from build123d import *

# Parameters (mm, degrees)
F0_W      = 228.6
F0_H      = 228.6
F1_DEPTH  = 38.1
F2_W      = 152.4
F2_H      = 152.4
F3_DEPTH  = 38.1
F4_W      = 38.1
F4_H      = 38.1
F5_DEPTH  = 1143
F6_W      = 228.6
F6_H      = 228.6
F7_DEPTH  = 38.1
F8_W      = 152.4
F8_H      = 152.4
F9_DEPTH  = 38.1
F10_W     = 38.1
F10_H     = 38.1
F11_DEPTH = 342.9
F12_W     = 38.1
F12_H     = 38.1
F13_DEPTH = 342.9
F14_R     = 6.35
F15_DEPTH = 0.254
F16_R     = 6.35
F17_DEPTH = 0.254
F18_R     = 6.35
F19_DEPTH = 0.254


with BuildPart() as f1:
    # F0 (on Top) → F1 (new body)
    with BuildSketch(Plane.XY):
        Rectangle(F0_W, F0_H)
    extrude(amount=-F1_DEPTH)

    # F2 (on face) → F3 (cut)
    with BuildSketch(Plane.XY):
        Rectangle(F2_W, F2_H)
    extrude(amount=-F3_DEPTH, mode=Mode.SUBTRACT)

    # F4 (on face) → F5 (join)
    with BuildSketch(Plane.XY):
        with Locations((-95.25, 95.25)):
            Rectangle(F4_W, F4_H)
        with Locations((95.25, 95.25)):
            Rectangle(F4_W, F4_H)
        with Locations((95.25, -95.25)):
            Rectangle(F4_W, F4_H)
        with Locations((-95.25, -95.25)):
            Rectangle(F4_W, F4_H)
    extrude(amount=F5_DEPTH)

    # F6 (on face) → F7 (join)
    with BuildSketch(Plane.XY.offset(1143)):
        Rectangle(F6_W, F6_H)
    extrude(amount=F7_DEPTH)

    # F8 (on face) → F9 (cut)
    with BuildSketch(Plane.XY.offset(1181.1)):
        Rectangle(F8_W, F8_H)
    extrude(amount=-F9_DEPTH, mode=Mode.SUBTRACT)

    # F10 (on face) → F11 (join)
    with BuildSketch(Plane(origin=(0, 0, 1143), x_dir=(1, 0, 0), z_dir=(0, 0, -1))):
        with Locations((95.25, 57.15)):
            Rectangle(F10_W, F10_H)
        with Locations((95.25, -57.15)):
            Rectangle(F10_W, F10_H)
    extrude(amount=F11_DEPTH)

    # F12 (on face) → F13 (join)
    with BuildSketch(Plane(origin=(0, 0, 1143), x_dir=(1, 0, 0), z_dir=(0, 0, -1))):
        with Locations((-95.25, -57.15)):
            Rectangle(F12_W, F12_H)
        with Locations((-95.25, 57.15)):
            Rectangle(F12_W, F12_H)
    extrude(amount=F13_DEPTH)

    # F14 (on face) → F15 (join)
    with BuildSketch(Plane(origin=(-114.3, 0, 0), x_dir=(0, -1, 0), z_dir=(-1, 0, 0))):
        with Locations((-95.25, -19.05)):
            Circle(F14_R)
        with Locations((95.25, -19.05)):
            Circle(F14_R)
    extrude(amount=F15_DEPTH)

    # F16 (on face) → F17 (cut)
    with BuildSketch(Plane.YZ.offset(-76.2)):
        with Locations((-57.15, 819.15)):
            Circle(F16_R)
        with Locations((57.15, 819.15)):
            Circle(F16_R)
    extrude(amount=-F17_DEPTH, mode=Mode.SUBTRACT)

    # F18 (on face) → F19 (cut)
    with BuildSketch(Plane(origin=(76.2, 0, 0), x_dir=(0, -1, 0), z_dir=(-1, 0, 0))):
        with Locations((-57.15, 819.15)):
            Circle(F18_R)
        with Locations((57.15, 819.15)):
            Circle(F18_R)
    extrude(amount=-F19_DEPTH, mode=Mode.SUBTRACT)


solid = f1.part
Verification items for the finished model (mm, model axes). A direction names the side the tool comes from. Coordinates: 2 decimals unless noted, no trailing zeros. Write each loop counter-clockwise with the first axis right and the second up, starting at its lowest first coordinate (ties: lowest second). Pieces come first, ordered by that corner, then holes. Notation, with made-up numbers: M 38.25,42 L 84.25,42 A29 cw 84.25,80 Z; hole C 43.25,69 d8. An arc over 180 degrees is marked long. Use a Markdown table: item, result.
Q1. Set-up check for faces 4 (the face through (95, 76.2, 394)), 5 (the face through (-1, -95, 0)), 6 (the face through (76.2, -1, -19)): record each of +Z, -Z, +X, -X, +Y, -Y from which the full face is reachable in a straight line by a thin tool's end or side.
Reply:
| item | result |
|---|---|
| face 4 | +X, -X |
| face 5 | +Y, -Y |
| face 6 | +Z, -Z |
Q2. Sectioned sample at A-A, the plane y = 9.5. Record the boundary of the cut face in (x, z).
Reply:
| item | result |
|---|---|
| outline | M -114.3,-38.1 L -76.2,-38.1 L -76.2,0 L -114.3,0 Z; M -114.3,1143 L -76.2,1143 L -76.2,1181.1 L -114.3,1181.1 Z; M 76.2,-38.1 L 114.3,-38.1 L 114.3,0 L 76.2,0 Z; M 76.2,1143 L 114.3,1143 L 114.3,1181.1 L 76.2,1181.1 Z |
Q3. Thickness scan on line 1 (Z direction, x = 76.4, y = 57.15); line 2 (Y direction, x = 76.3, z = 819.15); line 3 (Z direction, x = -17, y = -87). Record the ranges inside material, lowest first.
Reply:
| item | result |
|---|---|
| line 1 | z = -38.1 to 0, 800.1 to 812.8, 825.5 to 1181.1 |
| line 2 | y = -114.3 to -63.5, -50.8 to -38.1, 38.1 to 50.8, 63.5 to 114.3 |
| line 3 | z = -38.1 to 0, 1143 to 1181.1 |
Q4. Draft check along Y on faces 1 (the face through (-2, 78, 1181.1)), 2 (the face through (-1, 76.2, -19)), 3 (the face through (-96, 1, 0)). Enter one of: +Y half, -Y half, draft (parallel to the pull), parting line (faces both ways), or undercut.
Reply:
| item | result |
|---|---|
| face 1 | draft |
| face 2 | undercut |
| face 3 | undercut |
Q5. Go/stop test with a flat-tipped pin: P1, Ø6.5, axis at y = -56.5, z = 820.5, coming from the -X side. Record where the tip stops, or that it passes through.
Reply:
| item | result |
|---|---|
| P1 | stops at x = -114.3 |
